```python
from build123d import *

# Parameters (mm, degrees)
SKETCH1_W           = 175.26
SKETCH1_H           = 12.7
BOSS_EXTRUDE1_DEPTH = 96.8375
SKETCH2_W           = 5.08
SKETCH2_H           = 6.35
CUT_EXTRUDE1_DEPTH  = 213.67191875
CUT_EXTRUDE2_DEPTH  = 6.35
SKETCH5_W           = 15.875
SKETCH5_H           = 58.7375
CUT_EXTRUDE4_DEPTH  = 132.216646453
FILLET1_R           = 3.175


with BuildPart() as part:
    # Sketch1 → Boss-Extrude1 (new, symmetric)
    with BuildSketch(Plane(origin=(0, 0, 0), x_dir=(0, 0, -1), z_dir=(1, 0, 0))):
        Rectangle(SKETCH1_W, SKETCH1_H)
    extrude(amount=BOSS_EXTRUDE1_DEPTH, both=True)

    # Sketch2 → Cut-Extrude1 (cut, through all)
    with BuildSketch(Plane(origin=(96.8375, 0, 0), x_dir=(0, 0, -1), z_dir=(1, 0, 0))):
        with Locations((-85.09, -3.175)):
            Rectangle(SKETCH2_W, SKETCH2_H)
        with Locations((85.09, -3.175)):
            Rectangle(SKETCH2_W, SKETCH2_H)
    extrude(amount=-CUT_EXTRUDE1_DEPTH, mode=Mode.SUBTRACT)

    # Sketch3 → Cut-Extrude2 (cut)
    with BuildSketch(Plane(origin=(0, -6.35, 0), x_dir=(1, 0, 0), z_dir=(0, 1, 0))):
        with BuildLine():
            Line((28.448, 11.2395), (41.402, 11.2395))
            ThreePointArc((41.402, 11.2395), (44.704, 7.9375), (41.402, 4.6355))
            Line((41.402, 4.6355), (41.402, -4.6355))
            ThreePointArc((41.402, -4.6355), (44.704, -7.9375), (41.402, -11.2395))
            Line((41.402, -11.2395), (28.448, -11.2395))
            ThreePointArc((28.448, -11.2395), (25.146, -7.9375), (28.448, -4.6355))
            Line((28.448, -4.6355), (28.448, 4.6355))
            ThreePointArc((28.448, 4.6355), (25.146, 7.9375), (28.448, 11.2395))
        make_face()
        with BuildLine():
            Line((-22.352, 11.2395), (-9.398, 11.2395))
            ThreePointArc((-9.398, 11.2395), (-6.096, 7.9375), (-9.398, 4.6355))
            Line((-9.398, 4.6355), (-9.398, -4.6355))
            ThreePointArc((-9.398, -4.6355), (-6.096, -7.9375), (-9.398, -11.2395))
            Line((-9.398, -11.2395), (-22.352, -11.2395))
            ThreePointArc((-22.352, -11.2395), (-25.654, -7.9375), (-22.352, -4.6355))
            Line((-22.352, -4.6355), (-22.352, 4.6355))
            ThreePointArc((-22.352, 4.6355), (-25.654, 7.9375), (-22.352, 11.2395))
        make_face()
    extrude(amount=CUT_EXTRUDE2_DEPTH, mode=Mode.SUBTRACT)

    # Sketch5 → Cut-Extrude4 (cut, through all)
    with BuildSketch(Plane(origin=(0, 6.35, 0), x_dir=(1, 0, 0), z_dir=(0, 1, 0))):
        with Locations((9.525, -48.41875)):
            Rectangle(SKETCH5_W, SKETCH5_H)
        with Locations((9.525, 48.41875)):
            Rectangle(SKETCH5_W, SKETCH5_H)
    extrude(amount=-CUT_EXTRUDE4_DEPTH, mode=Mode.SUBTRACT)

    # Fillet1
    fillet1_edges = [part.edges().sort_by_distance(p)[0] for p in [
        (1.5875, 0, -19.05),
        (1.5875, 0, -77.7875),
        (17.4625, 0, -77.7875),
        (17.4625, 0, -19.05),
        (1.5875, 0, 77.7875),
        (1.5875, 0, 19.05),
        (17.4625, 0, 19.05),
        (17.4625, 0, 77.7875),
    ]]
    fillet(fillet1_edges, radius=FILLET1_R)


solid = part.part
```
CAD build for the part. Positions are in the model's coordinates, mm. A direction names the side the tool comes from. Give positions to 0.01 mm unless a question says otherwise; leave off trailing zeros. Write each loop counter-clockwise with the first axis right and the second up, starting at its lowest first coordinate (ties: lowest second). Pieces come first, ordered by that corner, then holes. Notation, with made-up numbers: M -9.5,-25 L 11.5,-25 A20 cw 11.5,6 Z; hole C 74,51.5 d4. An arc over 180 degrees is marked long. Return JSON: item names as keys, results as strings. Group by question number.
(1) 3-axis set-ups, long thin cutter, end or side, ignore diameter. For faces 1 (the face through (25.147, -3.219, 8.01)), 2 (the face through (1, 6.35, 1)), 3 (the face through (17.462, 0, -48)): which of +Z, -Z, +X, -X, +Y, -Y reach the whole face in a straight line?
(2) Mould opens along Z. For faces 4 (the face through (1, 0, 85)), 5 (the face through (-16, -3, 11.24)), 6 (the face through (1, -3, 82.55)) say: pulls with the +Z half, pulls with the -Z half, needs draft (parallel to the pull), parting line crosses it, or undercut.
(3) Band-saw the part on A-A (x = 11). Give the cut face in (y, z).
(4) Band-saw the part on D-D (y = 3.25). State how many separate pieces and enclosed holes the cut face has, and give its area (3 significant figures).
(5) Flat gauge pins, fed straight in: pin 1 Ø3 at (x, y) = (33.5, -3) entering from +Z; pin 2 Ø2.5 at (x, z) = (-26.5, 84.5) entering from -Y; pin 3 Ø3 at (x, y) = (24, -3.5) entering from -Z; pin 4 Ø21.5 at (x, z) = (-16.5, 1) entering from -Y. Where does each tip first touch, or does it go through?
(6) Band-saw the part on C-C (x = 37). Give the cut face in (y, z).
(7) Drill centre lines: L1, parallel to Z at x = 33, y = -4.5; L2, parallel to X at y = -5, z = -24; L3, parallel to Z at x = 74.5, y = -4.5. Where is each one in solid material? Low to high. Write a range as [from, to].
(8) Band-saw the part on B-B (z = -70). Give the cut face in (x, y).
Entries:
{
 "1": {"face 1": "-Y", "face 2": "+Z, -Z, +X, -X, +Y", "face 3": "+Y, -Y"},
 "2": {"face 4": "needs draft", "face 5": "undercut", "face 6": "pulls with the +Z half"},
 "3": {"outline": "M -6.35,-82.55 L 0,-82.55 L 0,-87.63 L 6.35,-87.63 L 6.35,-77.79 L -6.35,-77.79 Z; M -6.35,-19.05 L 6.35,-19.05 L 6.35,19.05 L -6.35,19.05 Z; M -6.35,77.79 L 6.35,77.79 L 6.35,87.63 L 0,87.63 L 0,82.55 L -6.35,82.55 Z"},
 "4": {"separate pieces": "1", "enclosed holes": "2", "area": "32,100 mm^2"},
 "5": {"pin 1": "stops at z = 82.55", "pin 2": "stops at y = 0", "pin 3": "stops at z = -82.55", "pin 4": "stops at y = -6.35"},
 "6": {"outline": "M -6.35,-82.55 L 0,-82.55 L 0,-87.63 L 6.35,-87.63 L 6.35,87.63 L 0,87.63 L 0,82.55 L -6.35,82.55 L -6.35,11.24 L 0,11.24 L 0,-11.24 L -6.35,-11.24 Z"},
 "7": {"L1": "z = [-82.55, -11.24], [11.24, 82.55]", "L2": "x = [-96.84, 1.59], [17.46, 96.84]", "L3": "z = [-82.55, 82.55]"},
 "8": {"outline": "M -96.84,-6.35 L 1.59,-6.35 L 1.59,6.35 L -96.84,6.35 Z; M 17.46,-6.35 L 96.84,-6.35 L 96.84,6.35 L 17.46,6.35 Z"}
}
